Geometry check sheet. Reference: drawing and pictorial views, mm from the part's lowest x, y, z. A direction names the side the tool comes from. Give positions to 0.01 mm unless a question says otherwise; leave off trailing zeros. Order: outer loops, then holes, each group sorted by start corner. A loop starts at its lowest first (then second) coordinate and runs counter-clockwise, first axis right, second up.
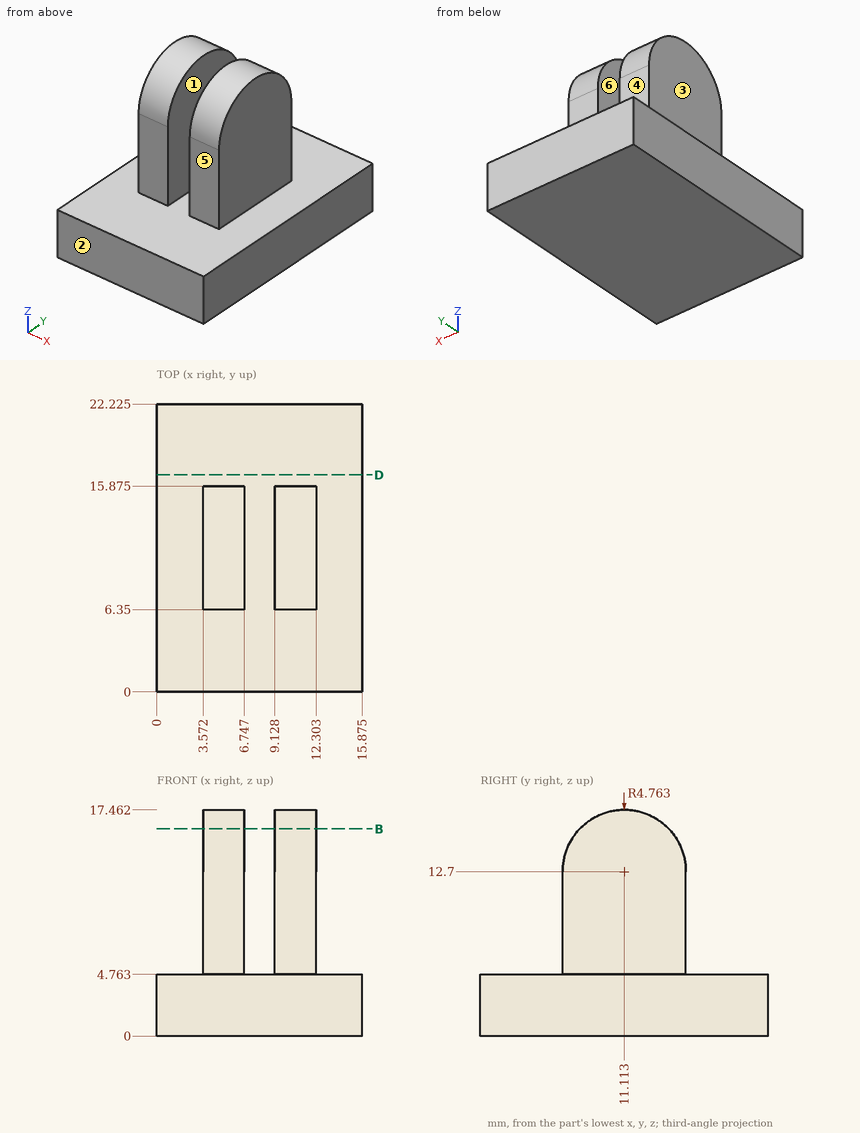
1) Section check B-B, the plane z = 16. Record the cut outline in (x, y).
Recorded:
outline: (3.57, 7.68) - (6.75, 7.68) - (6.75, 14.55) - (3.57, 14.55) - close; (9.13, 7.68) - (12.3, 7.68) - (12.3, 14.55) - (9.13, 14.55) - close
2) Material ranges on L1, parallel to X at y = 6.75, z = 6.75; L2, parallel to Z at x = 8.5, y = 18.5; L3, parallel to Z at x = 9.25, y = 13, recorded low to high.
Recorded:
L1: x = 3.57 to 6.75, 9.13 to 12.3
L2: z = 0 to 4.76
L3: z = 0 to 17.07
3) Depth check by flat-ended pin: pin 1 Ø4 at (y, z) = (6, 12.5) entering from -X; pin 2 Ø5 at (y, z) = (11, 8) entering from +X; pin 3 Ø3.5 at (x, z) = (5.5, 9) entering from +Y (1 decimal); pin 4 Ø4 at (y, z) = (11, 6) entering from -X. Enter the tip coordinate at first touch or a pass-through.
Recorded:
pin 1: stops at x = 3.57
pin 2: stops at x = 12.3
pin 3: stops at y = 15.9
pin 4: stops at x = 0
4) Section check D-D, the plane y = 16.75. Record the cut outline in (x, z) (1 decimal).
Recorded:
outline: (0, 0) - (15.9, 0) - (15.9, 4.8) - (0, 4.8) - close
5) Draft check along X on the marked faces 1, 2 and 3. Enter one of: +X half, -X half, draft (parallel to the pull), parting line (faces both ways), or undercut.
Recorded:
face 1: undercut
face 2: draft
face 3: -X half
6) Set-up check for the marked faces 4, 5 and 6: record each of +Z, -Z, +X, -X, +Y, -Y from which the full face is reachable in a straight line by a thin tool's end or side.
Recorded:
face 4: +Z, +X, -X, +Y
face 5: +Z, +X, -X, -Y
face 6: +Z, +Y, -Y
